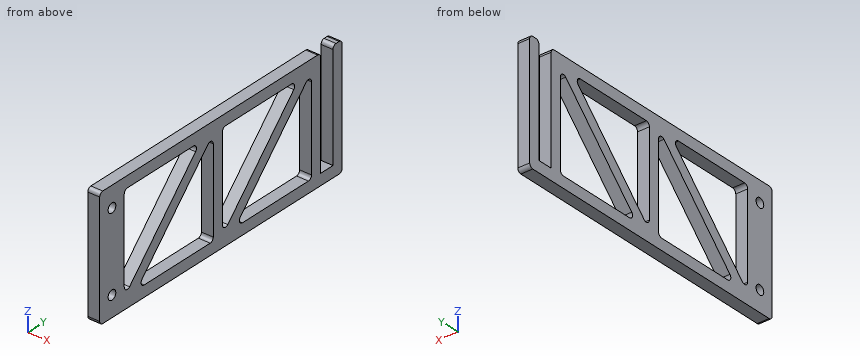
```python
from build123d import *

# Parameters (mm, degrees)
SKETCH1_W             = 32
SKETCH1_H             = 79
BOSS_EXTRUDE1_DEPTH   = 3.175
SKETCH2_W             = 29
SKETCH2_H             = 4
CUT_EXTRUDE1_DEPTH    = 3.175
F_2_5MM_DOWEL_HOLE1_D = 2.5
CUT_EXTRUDE2_DEPTH    = 3.175
FILLET2_R             = 1
FILLET3_R             = 1


with BuildPart() as part:
    # Sketch1 → Boss-Extrude1 (new body)
    with BuildSketch(Plane(origin=(0, 0, 0), x_dir=(0, 0, -1), z_dir=(1, 0, 0))):
        Rectangle(SKETCH1_W, SKETCH1_H)
    extrude(amount=BOSS_EXTRUDE1_DEPTH)

    # Sketch2 → Cut-Extrude1 (cut)
    with BuildSketch(Plane(origin=(3.175, 0, 0), x_dir=(0, 0, -1), z_dir=(1, 0, 0))):
        with Locations((-1.5, 34.5)):
            Rectangle(SKETCH2_W, SKETCH2_H)
    extrude(amount=-CUT_EXTRUDE1_DEPTH, mode=Mode.SUBTRACT)

    # Ø2.5mm Dowel Hole1 (through all)
    with Locations(Plane.ZY):
        with Locations((-10.5, -35.5), (10.5, -35.5)):
            Hole(F_2_5MM_DOWEL_HOLE1_D / 2)

    # Sketch8 → Cut-Extrude2 (cut)
    with BuildSketch(Plane(origin=(3.175, 0, 0), x_dir=(0, 0, -1), z_dir=(1, 0, 0))):
        Polygon((-13, -31.5), (13, -31.5), (-13, -6.649883213), align=None)
        Polygon((-13, -2.5), (13, -27.350116787), (13, -2.5), align=None)
        Polygon((-13, 0.5), (13, 0.5), (-13, 25.350116787), align=None)
        Polygon((-13, 29.5), (13, 4.649883213), (13, 29.5), align=None)
    extrude(amount=-CUT_EXTRUDE2_DEPTH, mode=Mode.SUBTRACT)

    # Fillet2
    fillet2_edges = [part.edges().sort_by_distance(p)[0] for p in [
        (1.5875, 32.5, 16),
        (1.5875, 36.5, 16),
        (1.5875, -39.5, -16),
        (1.5875, -39.5, 16),
        (1.5875, 39.5, 16),
        (1.5875, 39.5, -16),
    ]]
    fillet(fillet2_edges, radius=FILLET2_R)

    # Fillet3
    fillet3_edges = [part.edges().sort_by_distance(p)[0] for p in [
        (1.5875, -2.5, -13),
        (1.5875, -27.350116787, -13),
        (1.5875, -2.5, 13),
        (1.5875, 0.5, 13),
        (1.5875, 25.350116787, 13),
        (1.5875, 0.5, -13),
        (1.5875, 29.5, -13),
        (1.5875, 4.649883213, -13),
        (1.5875, 29.5, 13),
        (1.5875, -31.5, 13),
        (1.5875, -6.649883213, 13),
        (1.5875, -31.5, -13),
    ]]
    fillet(fillet3_edges, radius=FILLET3_R)


solid = part.part
```
Could you check a few things on this model? Use its own coordinates, in mm. Coordinates: 2 decimals unless noted, no trailing zeros. Write each loop counter-clockwise with the first axis right and the second up, starting at its lowest first coordinate (ties: lowest second). Pieces come first, ordered by that corner, then holes. Notation, with made-up numbers: (-20, -16) -> (-1, -16) arc R12 ccw to (-1, -5) -> close; hole circle Ø6 at (38, 87.25). An arc over 180 degrees is marked (long way). One line per question, with ' | ' between items. Start each with the question number.
1. If we section it at D-D (y = -10): Please give me the cut outline in (x, z) (3 decimals), and give its area (3 significant figures).
2. If we section it at C-C (x = 1.9): Count the separate pieces of the cut face and the enclosed holes in it, and give its area (3 significant figures).
3. If we section it at B-B (z = 1.5): Please give me the cut outline in (x, y) (3 decimals), and give its area (3 significant figures).
4. Please list where these lines run through material, in increasing order: line 1 along Y through (x, z) = (2.45, 5); line 2 along Z through (x, y) = (2.25, -12); line 3 along Y through (x, z) = (0.3, 3).
5. If we section it at A-A (y = -35.5): Please give me the cut outline in (x, z) (3 decimals).
Return value:
1) outline: (0, -16) -> (3.175, -16) -> (3.175, -13) -> (0, -13) -> close; (0, 5.153) -> (3.175, 5.153) -> (3.175, 9.495) -> (0, 9.495) -> close; (0, 13) -> (3.175, 13) -> (3.175, 16) -> (0, 16) -> close | area: 32.8 mm²
2) separate pieces: 1 | enclosed holes: 6 | area: 1,120 mm²
3) outline: (0, -39.5) -> (3.175, -39.5) -> (3.175, -31.5) -> (0, -31.5) -> close; (0, -17.641) -> (3.175, -17.641) -> (3.175, -13.491) -> (0, -13.491) -> close; (0, -2.5) -> (3.175, -2.5) -> (3.175, 0.5) -> (0, 0.5) -> close; (0, 14.359) -> (3.175, 14.359) -> (3.175, 18.509) -> (0, 18.509) -> close; (0, 29.5) -> (3.175, 29.5) -> (3.175, 32.5) -> (0, 32.5) -> close; (0, 36.5) -> (3.175, 36.5) -> (3.175, 39.5) -> (0, 39.5) -> close | area: 80.3 mm²
4) line 1: y = -39.5 to -31.5, -14.3 to -10.15, -2.5 to 0.5, 17.7 to 21.85, 29.5 to 32.5, 36.5 to 39.5 | line 2: z = -16 to -13, 3.06 to 7.4, 13 to 16 | line 3: y = -39.5 to -31.5, -16.21 to -12.06, -2.5 to 0.5, 15.79 to 19.94, 29.5 to 32.5, 36.5 to 39.5
5) outline: (0, -16) -> (3.175, -16) -> (3.175, -11.75) -> (0, -11.75) -> close; (0, -9.25) -> (3.175, -9.25) -> (3.175, 9.25) -> (0, 9.25) -> close; (0, 11.75) -> (3.175, 11.75) -> (3.175, 16) -> (0, 16) -> close
